Work out the finished part from the listing and answer in its coordinate system (mm). A direction names the side the tool comes from. Round coordinates to 2 decimals unless told otherwise and drop trailing zeros. Loops run counter-clockwise (first coordinate to the right, second up) from the corner with the lowest first, then second, coordinate; pieces in that order, holes last. Notation, with made-up numbers: M -1.75,76 L 18.25,76 A19 ccw 18.25,91 Z; hole C -39,23 d4. An arc over 180 degrees is marked long. One line per item, written item: value.
```python
from build123d import *

# Parameters (mm, degrees)
ESQUISSE2_R        = 0.3
BOSS_EXTRU_1_DEPTH = 2.5
ESQUISSE3_R        = 0.3
BOSS_EXTRU_2_DEPTH = 1
BOSS_EXTRU_3_DEPTH = 0.25
ESQUISSE5_R        = 0.6
BOSS_EXTRU_4_DEPTH = 0.2


with BuildPart() as part:
    # Esquisse1 → Révolution1 (revolve)
    with BuildSketch(Plane.XY, mode=Mode.PRIVATE) as r_volution1_sk:
        with BuildLine():
            Line((-2.5, 6.1), (-2.5, 1))
            Line((-2.5, 1), (-3, 1))
            Line((-3, 1), (-3, 0))
            Line((-3, 0), (0, 0))
            Line((0, 0), (0, 0.5))
            Line((0, 0.5), (-2.2, 0.5))
            Line((-2.2, 0.5), (-2.2, 6.1))
            ThreePointArc((-2.2, 6.1), (-1.555634919, 7.655634919), (0, 8.3))
            Line((0, 8.3), (0, 8.6))
            ThreePointArc((0, 8.6), (-1.767766953, 7.867766953), (-2.5, 6.1))
        make_face()
    revolve(r_volution1_sk.sketch.rotate(Axis((0, 0, 0), (0, 1, 0)), 270), axis=Axis((0, 0, 0), (0, 1, 0)))

    # Esquisse2 → Boss.-Extru.1 (add)
    with BuildSketch(Plane.XZ):
        with Locations(Location((-1.27, 0, 0), (0, 0, 90))):
            Circle(ESQUISSE2_R)
    extrude(amount=BOSS_EXTRU_1_DEPTH)

    # Esquisse3 → Boss.-Extru.2 (add)
    with BuildSketch(Plane.XZ):
        with Locations(Location((1.27, 0, 0), (0, 0, 90))):
            Circle(ESQUISSE3_R)
    extrude(amount=BOSS_EXTRU_2_DEPTH)

    # Esquisse4 → Boss.-Extru.3 (add, symmetric)
    with BuildSketch(Plane.XY):
        Polygon((-1.12, 4.2), (-0.610441672, 2.8), (0.32, 2.8), (0.32, 2.2), (-0.92, 2.2), (-0.92, 0), (-1.62, 0), (-1.62, 4.2), align=None)
        Polygon((-0.694328891, 4.2), (1.62, 4.2), (1.62, 0), (0.92, 0), (0.92, 3.2), (-0.330358657, 3.2), align=None)
    extrude(amount=BOSS_EXTRU_3_DEPTH, both=True)

    # Esquisse5 → Boss.-Extru.4 (add)
    with BuildSketch(Plane(origin=(0, 4.2, 0), x_dir=(1, 0, 0), z_dir=(0, 1, 0))):
        Circle(ESQUISSE5_R)
    extrude(amount=-BOSS_EXTRU_4_DEPTH)


solid = part.part
```
1) The mould has two halves that part along X. Classify faces 1 (the face through (-0.9, 0.49, -2.86)), 2 (the face through (-2, 1, -2)), 3 (the face through (1.3, 2.8, -0.25)): +X half, -X half, draft (parallel to the pull), parting line (faces both ways), or undercut.
Check values:
face 1: parting line
face 2: draft
face 3: undercut
2) Find section D-D (x = 0.75). Give the vertices of the cut face in (y, z).
Check values:
outline: M 0,-2.9 L 1,-2.9 L 1,-2.38 L 6.1,-2.38 A2.38 ccw 6.1,2.38 L 1,2.38 L 1,2.9 L 0,2.9 Z; M 3.2,-0.25 L 4.2,-0.25 L 4.2,0.25 L 3.2,0.25 Z; hole M 0.5,-2.07 L 6.1,-2.07 A2.07 ccw 6.1,2.07 L 0.5,2.07 Z
3) Find section A-A (y = 2). Give the vertices of the cut face in (x, z).
Check values:
outline: C 0,0 d5; M -1.62,-0.25 L -0.92,-0.25 L -0.92,0.25 L -1.62,0.25 Z; M 0.92,-0.25 L 1.62,-0.25 L 1.62,0.25 L 0.92,0.25 Z; hole C 0,0 d4.4
4) Find the intervals of material crossed by probe 1 along X at (y, z) = (2.1, 0); probe 2 along X at (y, z) = (2.65, 0); probe 3 along Y at (x, z) = (0.8, 0.15), in increasing order. Write a range as from..to.
Check values:
probe 1: -2.5..-2.2, -1.62..-0.92, 0.92..1.62, 2.2..2.5
probe 2: -2.5..-2.2, -1.62..0.32, 0.92..1.62, 2.2..2.5
probe 3: 0..0.5, 3.2..4.2, 8.14..8.46
5) Find section B-B (x = 0). Give the vertices of the cut face in (y, z).
Check values:
outline: M 0,-3 L 1,-3 L 1,-2.5 L 6.1,-2.5 A2.5 ccw 6.1,2.5 L 1,2.5 L 1,3 L 0,3 Z; M 2.2,-0.25 L 2.8,-0.25 L 2.8,0.25 L 2.2,0.25 Z; M 3.2,-0.25 L 4,-0.25 L 4,-0.6 L 4.2,-0.6 L 4.2,0.6 L 4,0.6 L 4,0.25 L 3.2,0.25 Z; hole M 0.5,-2.2 L 6.1,-2.2 A2.2 ccw 6.1,2.2 L 0.5,2.2 Z
6) For faces 4 (the face through (2.44, 3.51, 0.54)), 5 (the face through (0, 0.5, 0)), determine the directions among +Z, -Z, +X, -X, +Y, -Y from which every point of the face is accessible in a straight line to the end or side of a thin tool.
Check values:
face 4: +Y
face 5: none
7) Each of these flat-tipped pins is pushed along its axis until it touches: pin 1 (1.5 mm diameter, centred on y = 2, z = -0.5, fed in from +X); pin 2 (0.6 mm diameter, centred on x = -1.5, z = 0, fed in from +Y); pin 3 (1.6 mm diameter, centred on x = -0.5, y = 3, fed in from +Z). Where does it stop, or does it pass through?
Check values:
pin 1: x = 2.5
pin 2: y = 8.29
pin 3: z = 2.5
